Verification items for the finished model (mm, model axes). Face numbers are marked on the shaded views. A direction names the side the tool comes from. Coordinates: 2 decimals unless noted, no trailing zeros. Write each loop counter-clockwise with the first axis right and the second up, starting at its lowest first coordinate (ties: lowest second). Pieces come first, ordered by that corner, then holes.
```python
from build123d import *

# Parameters (mm, degrees)
F1_DEPTH  = 77.5
F2_W      = 7.5
F2_H      = 7.5
F3_DEPTH  = 5
F6_DEPTH  = 2.25
F7_DEPTH  = 2.25
F10_DEPTH = 2.25
F11_DEPTH = 2.25


with BuildPart() as f1:
    # F0 (on Front) → F1 (new body)
    with BuildSketch(Plane.XZ):
        with BuildLine():
            ThreePointArc((-28, -6.6598297656), (-25.0710678119, -13.7308975774), (-18, -16.6598297656))
            Line((-18, -16.6598297656), (-12, -16.6598297656))
            ThreePointArc((-12, -16.6598297656), (-8.4644660941, -15.1953636715), (-7, -11.6598297656))
            Line((-7, -11.6598297656), (-7, -11.1598297656))
            ThreePointArc((-7, -11.1598297656), (-6.7071067812, -10.4527229844), (-6, -10.1598297656))
            Line((-6, -10.1598297656), (6, -10.1598297656))
            ThreePointArc((6, -10.1598297656), (6.7071067812, -10.4527229844), (7, -11.1598297656))
            Line((7, -11.1598297656), (7, -11.6598297656))
            ThreePointArc((7, -11.6598297656), (8.4644660941, -15.1953636715), (12, -16.6598297656))
            Line((12, -16.6598297656), (18, -16.6598297656))
            ThreePointArc((18, -16.6598297656), (25.0710678119, -13.7308975774), (28, -6.6598297656))
            Line((28, -6.6598297656), (28, -4.3337819374))
            ThreePointArc((28, -4.3337819374), (25.933271977, 1.7541730344), (20.5873608522, 5.3256985776))
            Line((20.5873608522, 5.3256985776), (0, 10.8401702344))
            Line((0, 10.8401702344), (-20.5873608522, 5.3256985776))
            ThreePointArc((-20.5873608522, 5.3256985776), (-25.933271977, 1.7541730344), (-28, -4.3337819374))
            Line((-28, -4.3337819374), (-28, -6.6598297656))
        make_face()
    extrude(amount=F1_DEPTH)

    # F2 (on face) → F3 (join)
    with BuildSketch(Plane.XZ.offset(77.5)):
        with Locations((-16.5, -4.9098297656)):
            Rectangle(F2_W, F2_H)
        with Locations((12.5, -4.9098297656)):
            Rectangle(F2_W, F2_H)
    extrude(amount=F3_DEPTH)

    # F4 (on face) → F6 (cut)
    with BuildSketch(Plane.XY.offset(-1.1598297656)):
        Polygon((-12.75, -77.5), (-17.25, -77.5), (-17.25, -80), (-12.75, -80.5), align=None)
    extrude(amount=-F6_DEPTH, mode=Mode.SUBTRACT)

    # F5 (on face) → F7 (cut)
    with BuildSketch(Plane.XY.offset(-1.1598297656)):
        Polygon((16.25, -77.5), (11.75, -77.5), (11.75, -80), (16.25, -80.5), align=None)
    extrude(amount=-F7_DEPTH, mode=Mode.SUBTRACT)

    # F8 (on face) → F10 (cut)
    with BuildSketch(Plane(origin=(0, 0, -8.6598297656), x_dir=(1, 0, 0), z_dir=(0, 0, -1))):
        Polygon((11.75, 80), (11.75, 77.5), (16.25, 77.5), (16.25, 80.5), align=None)
    extrude(amount=-F10_DEPTH, mode=Mode.SUBTRACT)

    # F9 (on face) → F11 (cut)
    with BuildSketch(Plane(origin=(0, 0, -8.6598297656), x_dir=(1, 0, 0), z_dir=(0, 0, -1))):
        Polygon((-17.25, 80), (-17.25, 77.5), (-12.75, 77.5), (-12.75, 80.5), align=None)
    extrude(amount=-F11_DEPTH, mode=Mode.SUBTRACT)


solid = f1.part
```
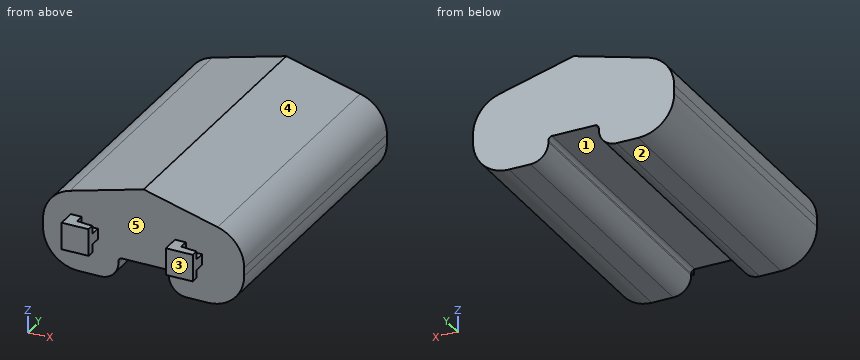
1. Sectioned sample at A-A, the plane y = -12. Record the boundary of the cut face in (x, z).
2. Tool access check on the marked faces 1 and 2. Record the directions out of +Z, -Z, +X, -X, +Y, -Y that give a thin tool (end or side, any length) a straight path to the whole face; none if there is none.
3. Draft check along X on the marked faces 3, 4 and 5. Enter one of: pulls with the +X half, pulls with the -X half, needs draft (parallel to the pull), parting line crosses it, or undercut.
4. Sectioned sample at B-B, the plane z = -13.25. Record the boundary of the cut face in (x, y).
5. Gauge pin test, flat ends, axial feed: P1, Ø0.9, axis at x = 13.5, y = -78.5, coming from the -Z side; P2, Ø1.5, axis at y = -80, z = -6, coming from the +X side; P3, Ø13, axis at x = -3, y = -46, coming from the -Z side. Record the tip position at first contact, or that the pin passes through.
6. Sectioned sample at D-D, the plane x = -19. Record the boundary of the cut face in (y, z), and give its area (3 significant figures).
7. Material ranges on L1, parallel to Y at x = -13.5, z = -0.75; L2, parallel to X at y = -67, z = -11.5; L3, parallel to X at y = -63.5, z = -12.25, recorded low to high.
8. Sectioned sample at C-C, the plane x = 13.5. Record the boundary of the cut face in (y, z), and give its area (3 significant figures).
Outcome:
1. outline: (-28, -6.66) arc R10 ccw to (-18, -16.66) - (-12, -16.66) arc R5 ccw to (-7, -11.66) - (-7, -11.16) arc R1 cw to (-6, -10.16) - (6, -10.16) arc R1 cw to (7, -11.16) - (7, -11.66) arc R5 ccw to (12, -16.66) - (18, -16.66) arc R10 ccw to (28, -6.66) - (28, -4.33) arc R10 ccw to (20.59, 5.33) - (0, 10.84) - (-20.59, 5.33) arc R10 ccw to (-28, -4.33) - close
2. face 1: -Z, +Y, -Y
2. face 2: -Z, +X, -X, +Y, -Y
3. face 3: needs draft
3. face 4: pulls with the +X half
3. face 5: undercut
4. outline: (-25.52, -77.5) - (-7.26, -77.5) - (-7.26, 0) - (-25.52, 0) - close; (7.26, -77.5) - (25.52, -77.5) - (25.52, 0) - (7.26, 0) - close
5. P1: stops at z = -6.41
5. P2: stops at x = 16.25
5. P3: stops at z = -15.99
6. outline: (-82.5, -8.66) - (-77.5, -8.66) - (-77.5, -16.61) - (0, -16.61) - (0, 5.75) - (-77.5, 5.75) - (-77.5, -1.16) - (-82.5, -1.16) - close
6. area: 1,770 mm2
7. L1: y = -77.5 to 0
7. L2: x = -26.75 to -7, 7 to 26.75
7. L3: x = -26.29 to -7.03, 7.03 to 26.29
8. outline: (-82.5, -8.66) - (-80.19, -8.66) - (-80.19, -6.41) - (-77.5, -6.41) - (-77.5, -16.66) - (0, -16.66) - (0, 7.22) - (-77.5, 7.22) - (-77.5, -3.41) - (-80.19, -3.41) - (-80.19, -1.16) - (-82.5, -1.16) - close
8. area: 1,880 mm2
